Check sheet for the modelled part. Datum: model origin and axes. Units: mm. A direction names the side the tool comes from. Round coordinates to 2 decimals unless told otherwise and drop trailing zeros. Write each loop counter-clockwise with the first axis right and the second up, starting at its lowest first coordinate (ties: lowest second). Pieces come first, ordered by that corner, then holes.
Item 1: Release check for a two-part mould opening along Z. For faces 4 (the flat face through (-9.6, 2, -19)), 5 (the flat face through (8, -2, -18.15)) record: pulls with the +Z half, pulls with the -Z half, needs draft (parallel to the pull), parting line crosses it, or undercut.
Item 2: Material ranges on line 1 along X through (y, z) = (1.5, -19.15); line 2 along Z through (x, y) = (3, -2); line 3 along X through (y, z) = (1.7, 0.85), recorded low to high.
Item 3: Section check A-A, the plane x = 0.5. Record the cut outline in (y, z), plus the area to 3 significant figures.
Item 4: Set-up check for faces 1 (the flat face through (7, 1, -3)), 2 (the flat face through (15.9, -2, -9)), 3 (the flat face through (-8, 0, -19)): record each of +Z, -Z, +X, -X, +Y, -Y from which the full face is reachable in a straight line by a thin tool's end or side.
Item 5: Section check C-C, the plane x = 22.4. Record the cut outline in (y, z).
Item 6: Depth check by flat-ended pin: pin 1 (0.8 mm diameter, centred on y = 2, z = -6.5, fed in from +X); pin 2 (2 mm diameter, centred on x = 22.5, y = 1, fed in from -Z); pin 3 (6 mm diameter, centred on x = -4.5, z = -3.5, fed in from +Y). Enter the tip coordinate at first touch or a pass-through.
Item 7: Section check B-B, the plane z = -19.15. Record the cut outline in (x, y), plus the area to 3 significant figures.
Item 8: Section check D-D, the plane y = -1.25. Record the cut outline in (x, z).
from build123d import *

# Parameters (mm, degrees)
SKETCH1_R           = 1.75
SKETCH1_W           = 15.9
SKETCH1_H           = 2.15
BASE_DEPTH          = 2.5
SKETCH3_W           = 17.9
SKETCH3_H           = 2.15
CUT_EXTRUDE1_DEPTH  = 2
SKETCH4_W           = 19.9
SKETCH4_H           = 28
SKETCH4_W_2         = 15.9
SKETCH4_H_2         = 2.15
BOSS_EXTRUDE1_DEPTH = 4.3
SKETCH5_W           = 12.9
SKETCH5_H           = 6.15
CUT_EXTRUDE2_DEPTH  = 1.5
SKETCH6_W           = 27.5
SKETCH6_H           = 0.9
BOSS_EXTRUDE2_DEPTH = 1.5
SKETCH6_3_W         = 27.5
SKETCH6_3_H         = 0.9
SKETCH6_3_W_2       = 28.4
BOSS_EXTRUDE3_DEPTH = 1.5


with BuildPart() as part:
    # Sketch1 → Base (new body)
    with BuildSketch(Plane(origin=(0, 0, 0), x_dir=(1, 0, 0), z_dir=(0, 1, 0))):
        Polygon((-2, 15.15), (-2, -4.85), (26.4, -4.85), (26.4, 3.15), (17.9, 3.15), (17.9, 23.15), (-9.6, 23.15), (-9.6, 15.15), align=None)
        with Locations(Location((-5.6, 19.15, 0), (0, 0, 270))):
            Circle(SKETCH1_R, mode=Mode.SUBTRACT)
        with Locations(Location((22.4, -0.85, 0), (0, 0, 270))):
            Circle(SKETCH1_R, mode=Mode.SUBTRACT)
        with Locations((7.95, 1.075)):
            Rectangle(SKETCH1_W, SKETCH1_H, mode=Mode.SUBTRACT)
        with Locations((7.95, 9.075)):
            Rectangle(SKETCH1_W, SKETCH1_H, mode=Mode.SUBTRACT)
        with Locations((7.95, 17.075)):
            Rectangle(SKETCH1_W, SKETCH1_H, mode=Mode.SUBTRACT)
    extrude(amount=BASE_DEPTH)

    # Sketch3 → Cut-Extrude1 (cut)
    with BuildSketch(Plane(origin=(0, 2.5, 0), x_dir=(1, 0, 0), z_dir=(0, 1, 0))):
        with Locations((7.95, 17.075)):
            Rectangle(SKETCH3_W, SKETCH3_H)
        with Locations((7.95, 9.075)):
            Rectangle(SKETCH3_W, SKETCH3_H)
        with Locations((7.95, 1.075)):
            Rectangle(SKETCH3_W, SKETCH3_H)
    extrude(amount=-CUT_EXTRUDE1_DEPTH, mode=Mode.SUBTRACT)

    # Sketch4 → Boss-Extrude1 (add)
    with BuildSketch(Plane.XZ):
        with Locations((7.95, -9.15)):
            Rectangle(SKETCH4_W, SKETCH4_H)
        with Locations((7.95, -17.075)):
            Rectangle(SKETCH4_W_2, SKETCH4_H_2, mode=Mode.SUBTRACT)
        with Locations((7.95, -9.075)):
            Rectangle(SKETCH4_W_2, SKETCH4_H_2, mode=Mode.SUBTRACT)
        with Locations((7.95, -1.075)):
            Rectangle(SKETCH4_W_2, SKETCH4_H_2, mode=Mode.SUBTRACT)
    extrude(amount=BOSS_EXTRUDE1_DEPTH)

    # Sketch5 → Cut-Extrude2 (cut)
    with BuildSketch(Plane(origin=(0, 2.5, 0), x_dir=(1, 0, 0), z_dir=(0, 1, 0))):
        with Locations((7.45, 17.075)):
            Rectangle(SKETCH5_W, SKETCH5_H)
        with Locations((7.45, 9.075)):
            Rectangle(SKETCH5_W, SKETCH5_H)
        with Locations((7.45, 1.075)):
            Rectangle(SKETCH5_W, SKETCH5_H)
    extrude(amount=-CUT_EXTRUDE2_DEPTH, mode=Mode.SUBTRACT)

    # Sketch6 → Boss-Extrude2 (add)
    with BuildSketch(Plane(origin=(0, 2.5, 0), x_dir=(1, 0, 0), z_dir=(0, 1, 0))):
        with Locations((4.15, 22.7)):
            Rectangle(SKETCH6_W, SKETCH6_H)
    extrude(amount=BOSS_EXTRUDE2_DEPTH)

    # Sketch6_3 → Boss-Extrude3 (add)
    with BuildSketch(Plane(origin=(0, 2.5, 0), x_dir=(1, 0, 0), z_dir=(0, 1, 0))):
        with Locations((4.15, 22.7)):
            Rectangle(SKETCH6_3_W, SKETCH6_3_H)
        with Locations((12.2, -4.4)):
            Rectangle(SKETCH6_3_W_2, SKETCH6_3_H)
    extrude(amount=BOSS_EXTRUDE3_DEPTH)


solid = part.part
Values found:
1. face 4: needs draft
1. face 5: undercut
2. line 1: x = -9.6 to -7.35, -3.85 to 1, 13.9 to 17.9
2. line 2: z = -23.15 to -18.15, -16 to -10.15, -8 to -2.15, 0 to 4.85
2. line 3: x = -2 to 1, 13.9 to 20.65, 24.15 to 26.4
3. outline: (-4.3, -23.15) - (4, -23.15) - (4, -22.25) - (2.5, -22.25) - (2.5, -18.15) - (-4.3, -18.15) - close; (-4.3, -16) - (2.5, -16) - (2.5, -10.15) - (-4.3, -10.15) - close; (-4.3, -8) - (2.5, -8) - (2.5, -2.15) - (-4.3, -2.15) - close; (-4.3, 0) - (2.5, 0) - (2.5, 3.95) - (4, 3.95) - (4, 4.85) - (-4.3, 4.85) - close
3. area: 149 mm2
4. face 1: +Y
4. face 2: +Y, -Y
4. face 3: +Z, -Z, -X, -Y
5. outline: (0, -3.15) - (2.5, -3.15) - (2.5, -0.9) - (0, -0.9) - close; (0, 2.6) - (2.5, 2.6) - (2.5, 3.95) - (4, 3.95) - (4, 4.85) - (0, 4.85) - close
6. pin 1: stops at x = 17.9
6. pin 2: stops at z = -3.15
6. pin 3: stops at y = 2.5
7. outline: (-9.6, 0) - (-7.35, 0) - (-7.35, 2.5) - (-9.6, 2.5) - close; (-3.85, 0) - (-2, 0) - (-2, -4.3) - (17.9, -4.3) - (17.9, 2.5) - (13.9, 2.5) - (13.9, 1) - (1, 1) - (1, 2.5) - (-3.85, 2.5) - close
7. area: 126 mm2
8. outline: (-2, -23.15) - (17.9, -23.15) - (17.9, 4.85) - (-2, 4.85) - close; hole (0, -18.15) - (15.9, -18.15) - (15.9, -16) - (0, -16) - close; hole (0, -10.15) - (15.9, -10.15) - (15.9, -8) - (0, -8) - close; hole (0, -2.15) - (15.9, -2.15) - (15.9, 0) - (0, 0) - close
